Autodesk Inventor part; units mm, degrees
ref_plane "YZ Plane" through (0, 0, 0) normal (1, 0, 0) x (0, 1, 0)
ref_plane "XZ Plane" through (0, 0, 0) normal (0, 1, 0) x (-1, 0, 0)
ref_plane "XY Plane" through (0, 0, 0) normal (0, 0, 1) x (1, 0, 0)
sketch "Sketch9" plane through (0, 0, 0) normal (0, 0, 1) x (1, 0, 0)
  circle A0 centre (-9.3, -6.3) radius 2
  circle A1 centre (10.6, 6.6) radius 2
  line L0 (3.75, -3.75) -> (-3.75, -3.75) construction
  line L1 (-3.75, -3.75) -> (-3.75, 3.75) construction
  line L2 (-3.75, 3.75) -> (3.75, 3.75) construction
  line L3 (3.75, 3.75) -> (3.75, -3.75) construction
  line L4 (3.75, -3.75) -> (-3.75, 3.75) construction
  line L5 (-3.75, -3.75) -> (3.75, 3.75) construction
  line L6 (-4.95, -3.125) -> (-6.85, -3.125) construction
  line L7 (-6.85, -3.125) -> (-6.85, -1.175) construction
  line L8 (-6.85, -1.175) -> (-4.95, -1.175) construction
  line L9 (-4.95, -1.175) -> (-4.95, -3.125) construction
  line L10 (-4.95, -3.125) -> (-6.85, -1.175) construction
  line L11 (-6.85, -3.125) -> (-4.95, -1.175) construction
  line L12 (2.575, -4.925) -> (-0.575, -4.925) construction
  line L13 (-0.575, -4.925) -> (-0.575, -8.075) construction
  line L14 (-0.575, -8.075) -> (2.575, -8.075) construction
  line L15 (2.575, -8.075) -> (2.575, -4.925) construction
  line L16 (2.575, -4.925) -> (-0.575, -8.075) construction
  line L17 (-0.575, -4.925) -> (2.575, -8.075) construction
  line L18 (12.3232, 5.5848) -> (4.7232, -7.3152)
  arc A2 (3, -8.3) -> (4.7232, -7.3152) centre (3, -6.3) ccw
  line L19 (3, -8.3) -> (-9.3, -8.3)
  line L20 (-11.2363, -5.7994) -> (-7.5137, 8.5994)
  arc A3 (-7.5137, 8.5994) -> (-7.45, 9.1) centre (-9.45, 9.1) ccw
  line L21 (-7.45, 9.1) -> (-7.45, 10.1)
  line L22 (-7.45, 10.1) -> (4, 10.1)
  arc A4 (4, 10.1) -> (4.9131, 9.1038) centre (5, 10.1) ccw
  line L23 (4.9131, 9.1038) -> (10.7738, 8.5924)
  line L24 (3.25, -4.25) -> (-3.25, -4.25)
  line L25 (-4.25, -3.25) -> (-4.25, 3.25)
  line L26 (-3.25, 4.25) -> (3.25, 4.25)
  line L27 (4.25, 3.25) -> (4.25, -3.25)
  arc A5 (3.25, -4.25) -> (4.25, -3.25) centre (3.25, -3.25) ccw
  arc A6 (-4.25, -3.25) -> (-3.25, -4.25) centre (-3.25, -3.25) ccw
  arc A7 (-3.25, 4.25) -> (-4.25, 3.25) centre (-3.25, 3.25) ccw
  arc A8 (4.25, 3.25) -> (3.25, 4.25) centre (3.25, 3.25) ccw
  line L28 (1.7, 7.8) -> (-2.3, 7.8) construction
  line L29 (-2.3, 7.8) -> (-2.3, 5) construction
  line L30 (-2.3, 5) -> (1.7, 5) construction
  line L31 (1.7, 5) -> (1.7, 7.8) construction
  line L32 (1.7, 7.8) -> (-2.3, 5) construction
  line L33 (-2.3, 7.8) -> (1.7, 5) construction
  line L34 (-4.25, 3.25) -> (-4.25, 7.2)
  arc A9 (-3.25, 8.2) -> (-4.25, 7.2) centre (-3.25, 7.2) ccw
  line L35 (-3.25, 8.2) -> (3.25, 8.2)
  arc A10 (4.25, 7.2) -> (3.25, 8.2) centre (3.25, 7.2) ccw
  line L36 (4.25, 7.2) -> (4.25, 3.25)
  line L37 (-5.15, -3.4) -> (-6.65, -3.4)
  line L38 (-7.15, -2.9) -> (-7.15, -1.4)
  line L39 (-6.65, -0.9) -> (-5.15, -0.9)
  line L40 (-4.65, -1.4) -> (-4.65, -2.9)
  arc A11 (-5.15, -3.4) -> (-4.65, -2.9) centre (-5.15, -2.9) ccw
  arc A12 (-4.65, -1.4) -> (-5.15, -0.9) centre (-5.15, -1.4) ccw
  arc A13 (-6.65, -0.9) -> (-7.15, -1.4) centre (-6.65, -1.4) ccw
  arc A14 (-7.15, -2.9) -> (-6.65, -3.4) centre (-6.65, -2.9) ccw
  line L41 (2.5, -8.3) -> (-0.5, -8.3)
  line L42 (-1, -7.8) -> (-1, -5.2)
  line L43 (-0.5, -4.7) -> (2.5, -4.7)
  line L44 (3, -5.2) -> (3, -7.8)
  arc A15 (2.5, -8.3) -> (3, -7.8) centre (2.5, -7.8) ccw
  arc A16 (3, -5.2) -> (2.5, -4.7) centre (2.5, -5.2) ccw
  arc A17 (-0.5, -4.7) -> (-1, -5.2) centre (-0.5, -5.2) ccw
  arc A18 (-1, -7.8) -> (-0.5, -8.3) centre (-0.5, -7.8) ccw
  circle A19 centre (-7.6029, -4.1225) radius 1.05 construction
  line L45 (-9.3, -6.3) -> (-6.65, -2.9) construction
  line L46 (-7.4312, -5.5876) -> (-9.0655, -4.3138)
  line L47 (-4.25, 10.1) -> (-4.25, 7.2)
  line L48 (-7.45, 9.1) -> (-7.45, 6.6)
  arc A20 (-7.45, 6.6) -> (-6.95, 6.1) centre (-6.95, 6.6) ccw
  line L49 (-6.95, 6.1) -> (-4.75, 6.1)
  arc A21 (-4.75, 6.1) -> (-4.25, 6.6) centre (-4.75, 6.6) ccw
  point P0 (0, 0)
  point P1 (0, 0)
  point P2 (-5.9, -2.15)
  point P3 (1, -6.5)
  point P4 (0, 0)
  point P5 (0, -4.25)
  point P6 (0, 0)
  point P7 (-4.25, 0)
  point P8 (-0.3, 6.4)
  point P9 (1, -4.925)
  point P10 (1, -4.7)
  point P11 (-1, -6.5)
  point P12 (-0.575, -6.5)
  point P13 (-5.9, -3.4)
  point P14 (-5.9, -3.125)
  point P15 (-4.65, -2.15)
  point P16 (-4.95, -2.15)
  dimension "d71" = 4
  dimension "d72" = 19.9
  dimension "d73" = 12.9
  dimension "d74" = 9.3
  dimension "d75" = 6.3
  dimension "d76" = 7.5
  dimension "d77" = 5.9
  dimension "d78" = 2.15
  dimension "d79" = 1.9
  dimension "d80" = 1.95
  dimension "d81" = 6.5
  dimension "d82" = 1
  dimension "d83" = 3.15
  dimension "d95" = 2
  dimension "d96" = 3
  dimension "d97" = 10.1
  dimension "d103" = 1
  dimension "d104" = 8.5
  dimension "d107" = 6.4
  dimension "d108" = 2.8
  dimension "d109" = 4
  dimension "d110" = 0.3
  dimension "d111" = 1.8
  dimension "d114" = 0.5
  dimension "d115" = 0.5
  dimension "d116" = 4
  dimension "d117" = 2.5
  dimension "d118" = 2.5
  dimension "d119" = 2.1
  dimension "d120" = 1.7107
  dimension "d125" = 1
  dimension "d127" = 1
  dimension "d128" = 4
  dimension "d129" = 3.2
  dimension "d130" = 4
extrude "Extrusion7" add sketch "Sketch9" along normal blind 3.5 and the other way blind 1 contours A0 L46 | A1 picked at (-9.5, -5.1238)
sketch "Sketch10" plane through (10.6, 6.6, 3.5) normal (0, 0, 1) x (1, 0, 0)
  arc A0 (-19.6655, -10.9138) -> (-18.0312, -12.1876) centre (-19.9, -12.9) ccw
  circle A1 centre (0, 0) radius 2
  line L0 (-18.0312, -12.1876) -> (-19.6655, -10.9138)
  point P0 (-10.6, -6.6)
hole "Hole3" at (10.6, 6.6, 3.5) at (-9.3, -6.3, 3.5) direction (0, 0, -1) diameter 1.567 end through all
extrude "Extrusion8" add sketch "Sketch9" against normal up to surface (1 mm away) contours A0 L20 A3 L48 A20 L49 A21 L34 L25 A6 L24 A5 L27 L36 A10 L35 A9 L47 L22 A4 L23 A1 L18 A2 L19 A15 L44 A16 L43 A17 L42 A18 | L46 A0 | A18 L42 A17 L43 A16 L44 A15 L19 | L21 L22 L47 L34 A21 L49 A20 L48 | A9 L35 A10 L36 A8 L26 A7 L34 | A7 L26 A8 L27 A5 L24 A6 L25 | L37 A14 L38 A13 L39 A12 L40 A11 picked at (-8.1343, -4.9223)
extrude "Extrusion9" add sketch "Sketch9" along normal blind 0.5 contours A0 L20 A3 L48 A20 L49 A21 L34 L25 A6 L24 A5 L27 L36 A10 L35 A9 L47 L22 A4 L23 A1 L18 A2 L19 A15 L44 A16 L43 A17 L42 A18 | L46 A0 | A18 L42 A17 L43 A16 L44 A15 L19 | L21 L22 L47 L34 A21 L49 A20 L48 | A9 L35 A10 L36 A8 L26 A7 L34 | L37 A14 L38 A13 L39 A12 L40 A11 picked at (-8.1343, -4.9223)
extrude "Extrusion10" add sketch "Sketch9" along normal blind 1.4 contours A0 L20 A3 L48 A20 L49 A21 L34 L25 A6 L24 A5 L27 L36 A10 L35 A9 L47 L22 A4 L23 A1 L18 A2 L19 A15 L44 A16 L43 A17 L42 A18 | L46 A0 | A18 L42 A17 L43 A16 L44 A15 L19 | L21 L22 L47 L34 A21 L49 A20 L48 | L37 A14 L38 A13 L39 A12 L40 A11 picked at (-8.1343, -4.9223)
extrude "Extrusion11" add sketch "Sketch9" along normal blind 2.27 contours A18 L42 A17 L43 A16 L44 A15 L19
extrude "Extrusion12" add sketch "Sketch9" along normal blind 2.15 contours L37 A14 L38 A13 L39 A12 L40 A11
extrude "Extrusion13" add sketch "Sketch9" along normal blind 2.3 contours L21 L22 L47 L34 A21 L49 A20 L48
sketch "Sketch11" plane through (-7.45, 10.1, -1) normal (0, 1, 0) x (1, 0, 0)
  line L0 (0, 0) -> (0, -3.3)
  line L1 (3.2, -3.3) -> (0, -3.3)
  line L2 (3.2, -2.4) -> (3.2, -3.3)
  line L3 (11.45, -2.4) -> (3.2, -2.4)
  line L4 (11.45, 0) -> (11.45, -2.4)
  line L5 (0, 0) -> (11.45, 0)
  line L6 (0, 0) -> (11.45, 0) construction
  line L7 (0, 0) -> (3.2, -3.3) construction
  point P0 (7.45, -1)
  point P1 (1.6, -1.65)
hole "Hole4" at (-5.85, 10.1, 0.65) direction (0, -1, 0) diameter 1.221 depth 3 tip angle 118
equation "\"SilPad\" = 0.35"
properties part number "EPS_RegulatorHeatsink-A" material "Aluminum 6061"
Here's how the part is built. I have some questions about the finished solid (model axes, mm). A direction names the side the tool comes from. Round coordinates to 2 decimals unless told otherwise and drop trailing zeros. Write each loop counter-clockwise with the first axis right and the second up, starting at its lowest first coordinate (ties: lowest second). Pieces come first, ordered by that corner, then holes.
1. I need wall thicknesses on L1, parallel to Y at x = 0.25, z = 0.4; L2, parallel to Y at x = 2.75, z = 1.15; L3, parallel to Z at x = -5.85, y = 8.7. Which ranges of each line are inside material? Lowest first, please.
2. If we mould it in two halves opening along Y, with no side actions, what happens to faces 5 (the flat face through (-6, 6.1, 2)), 6 (the flat face through (-6, -2, 2.15)), 7 (the cylindrical face through (4, -8.03, 0.18))? For each: released by +Y, released by -Y, zero draft, split by the parting line, or undercut.
3. Suppose I cut it at B-B (x = 0). List the corners of the cut face in (y, z) for me, and give its area (3 significant figures).
4. Suppose I cut it at D-D (y = -2.5). List the corners of the cut face in (x, z) for me.
5. For faces 1 (the cylindrical face through (-8.605, -6.662, 1.219)), 2 (the flat face through (-7.45, 9.5, 1)), 3 (the flat face through (0, 8.2, 1)), 4 (the flat face through (-1, -7, 2)), which set-ups out of +Z, -Z, +X, -X, +Y, -Y let a thin tool reach every point of the face, with its end or its side?
6. Will these pins go through, and if not, where does the flat tip stop? pin 1 Ø5.5 at (x, y) = (-2.5, -2) entering from +Z; pin 2 Ø4 at (x, y) = (1, 2) entering from +Z; pin 3 Ø2.5 at (x, y) = (-1.5, 5.5) entering from +Z.
7. Suppose I cut it at A-A (z = 1.75). List the corners of the cut face in (x, y) for me, and give its area (3 significant figures).
8. Suppose I cut it at C-C (y = -6.3). List the corners of the cut face in (x, z) for me, and give its area (3 significant figures).
Answer sheet:
1. L1: y = -8.3 to -4.25, 4.25 to 10.1
1. L2: y = -8.3 to -4.25, 8.2 to 10.1
1. L3: z = -1 to 0.04, 1.26 to 2.3
2. face 5: undercut
2. face 6: zero draft
2. face 7: released by -Y
3. outline: (-8.3, -1) - (10.1, -1) - (10.1, 1.4) - (8.2, 1.4) - (8.2, 0.5) - (4.25, 0.5) - (4.25, 0) - (-4.25, 0) - (-4.25, 1.4) - (-4.7, 1.4) - (-4.7, 2.27) - (-8.3, 2.27) - close
3. area: 31.8 mm2
4. outline: (-10.38, -1) - (7.56, -1) - (7.56, 1.4) - (4.25, 1.4) - (4.25, 0) - (-4.25, 0) - (-4.25, 1.4) - (-4.65, 1.4) - (-4.65, 2.15) - (-7.15, 2.15) - (-7.15, 1.4) - (-10.38, 1.4) - close
5. face 1: +Z, -Z
5. face 2: +Z, -X, +Y
5. face 3: +Z
5. face 4: +Z, +Y, -Y
6. pin 1: stops at z = 2.15
6. pin 2: stops at z = 0
6. pin 3: stops at z = 0.5
7. outline: (-9.07, -4.31) arc R2 ccw (long way) to (-7.43, -5.59) - close; (-7.45, 6.6) arc R0.5 ccw to (-6.95, 6.1) - (-4.75, 6.1) arc R0.5 ccw to (-4.25, 6.6) - (-4.25, 10.1) - (-7.45, 10.1) - close; (-7.15, -2.9) arc R0.5 ccw to (-6.65, -3.4) - (-5.15, -3.4) arc R0.5 ccw to (-4.65, -2.9) - (-4.65, -1.4) arc R0.5 ccw to (-5.15, -0.9) - (-6.65, -0.9) arc R0.5 ccw to (-7.15, -1.4) - close; (-1, -7.8) arc R0.5 ccw to (-0.5, -8.3) - (2.5, -8.3) arc R0.5 ccw to (3, -7.8) - (3, -5.2) arc R0.5 ccw to (2.5, -4.7) - (-0.5, -4.7) arc R0.5 ccw to (-1, -5.2) - close; circle Ø4 at (10.6, 6.6); hole circle Ø1.57 at (-9.3, -6.3); hole circle Ø1.57 at (10.6, 6.6)
7. area: 53.8 mm2
8. outline: (-11.3, -1) - (-10.08, -1) - (-10.08, 3.5) - (-11.3, 3.5) - close; (-8.52, -1) - (5.32, -1) - (5.32, 1.4) - (3, 1.4) - (3, 2.27) - (-1, 2.27) - (-1, 1.4) - (-7.3, 1.4) - (-7.3, 3.5) - (-8.52, 3.5) - close
8. area: 44.7 mm2
